Autodesk Inventor part; units mm, degrees
ref_plane "YZ Plane" through (0, 0, 0) normal (1, 0, 0) x (0, 1, 0)
ref_plane "XZ Plane" through (0, 0, 0) normal (0, 1, 0) x (-1, 0, 0)
ref_plane "XY Plane" through (0, 0, 0) normal (0, 0, 1) x (1, 0, 0)
sketch "Эскиз1" plane through (0, 0, 0) normal (0, 0, 1) x (1, 0, 0)
  line L0 (-30.974, -13.01) -> (30.974, -13.01)
  line L1 (30.974, -13.01) -> (30.974, 13.01)
  line L2 (30.974, 13.01) -> (-30.974, 13.01)
  line L3 (-30.974, 13.01) -> (-30.974, -13.01)
  line L4 (-30.974, -13.01) -> (30.974, 13.01) construction
  line L5 (30.974, -13.01) -> (-30.974, 13.01) construction
  point P0 (0, 0)
  dimension "d0" = 61.948
  dimension "d1" = 26.02
extrude "Выдавливание1" add sketch "Эскиз1" along normal blind 10
sketch "Эскиз2" plane through (30.974, -13.01, 0) normal (1, 0, 0) x (0, 0, -1)
  line L0 (0, 13.01) -> (-5, 13.01)
  circle A0 centre (-5, 13.01) radius 2
  dimension "d4" = 5
  dimension "d5" = 4
extrude "Выдавливание2" cut sketch "Эскиз2" against normal blind 10
pattern_linear "Прямоуг.массив1" count 3 spacing 8 along (0, 1, 0) of "Выдавливание2" first direction both ways yes
mirror "Зеркальное отражение1" about plane through (0, 0, 0) normal (1, 0, 0) of "Выдавливание2", "Прямоуг.массив1"
sketch "Эскиз3" plane through (0, 0, 0) normal (0, 0, -1) x (-1, 0, 0)
  line L0 (0, 0) -> (-20, 0)
  line L1 (-30.974, 13.01) -> (30.974, 13.01)
  line L2 (30.974, -13.01) -> (-30.974, -13.01)
  line L3 (-20, 13.01) -> (-25, 13.01)
  line L4 (-25, 13.01) -> (-25, -13.01)
  line L5 (-25, -13.01) -> (-20, -13.01)
  line L6 (-20, -13.01) -> (-20, 13.01)
  line L7 (-30.974, -13.01) -> (-30.974, 13.01)
  dimension "d11" = 20
  dimension "d12" = 5
extrude "Выдавливание3" add sketch "Эскиз3" along normal blind 10 contours L1 L6 L2 L4
sketch "Эскиз4" plane through (25, -13.01, 0) normal (1, 0, 0) x (0, 0, -1)
  line L0 (10, 26.02) -> (10, 0)
  line L1 (10, 13.01) -> (5, 13.01)
  circle A0 centre (5, 13.01) radius 2
  point P0 (0, 13.01)
  dimension "d16" = 5
  dimension "d17" = 4
extrude "Выдавливание4" cut sketch "Эскиз4" against normal blind 10
pattern_linear "Прямоуг.массив2" count 3 spacing 8 along (0, -1, 0) of "Выдавливание4" first direction both ways yes
mirror "Зеркальное отражение2" about plane through (0, 0, 0) normal (1, 0, 0) of "Выдавливание3", "Выдавливание4", "Прямоуг.массив2"
sketch "Эскиз5" plane through (0, 0, 10) normal (0, 0, 1) x (1, 0, 0)
  circle A0 centre (0, 0) radius 7.5
  dimension "d23" = 15
extrude "Выдавливание5" cut sketch "Эскиз5" against normal blind 23.75
sketch "Эскиз6" plane through (0, 0, 10) normal (0, 0, 1) x (1, 0, 0)
  circle A0 centre (0, 0) radius 5
  line L0 (-13.4261, 4.5029) -> (-16.9261, 4.5029)
  line L1 (-16.9261, 4.5029) -> (-16.9261, 11.4971)
  line L2 (-16.9261, 11.4971) -> (-13.4261, 11.4971)
  line L3 (-13.4261, 11.4971) -> (-13.4261, 4.5029)
  line L4 (-13.4261, -11.4971) -> (-16.9261, -11.4971)
  line L5 (-16.9261, -11.4971) -> (-16.9261, -4.5029)
  line L6 (-16.9261, -4.5029) -> (-13.4261, -4.5029)
  line L7 (-13.4261, -4.5029) -> (-13.4261, -11.4971)
  line L8 (-13.4261, -3.4971) -> (-16.9261, -3.4971)
  line L9 (-16.9261, -3.4971) -> (-16.9261, 3.4971)
  line L10 (-16.9261, 3.4971) -> (-13.4261, 3.4971)
  line L11 (-13.4261, 3.4971) -> (-13.4261, -3.4971)
  line L12 (10.5, 4.5029) -> (7, 4.5029)
  line L13 (7, 4.5029) -> (7, 11.4971)
  line L14 (7, 11.4971) -> (10.5, 11.4971)
  line L15 (10.5, 11.4971) -> (10.5, 4.5029)
  line L16 (10.5, -11.4971) -> (7, -11.4971)
  line L17 (7, -11.4971) -> (7, -4.5029)
  line L18 (7, -4.5029) -> (10.5, -4.5029)
  line L19 (10.5, -4.5029) -> (10.5, -11.4971)
  line L20 (7, 3.4971) -> (10.5, 3.4971)
  line L21 (10.5, 3.4971) -> (10.5, -3.4971)
  line L22 (10.5, -3.4971) -> (7, -3.4971)
  line L23 (7, -3.4971) -> (7, 3.4971)
  line L24 (17, -13.1) -> (17, 13.1)
  line L25 (17, 13.1) -> (-17, 13.1)
  line L26 (-17, 13.1) -> (-17, -13.1)
  line L27 (-17, -13.1) -> (17, -13.1)
extrude "Выдавливание6" cut sketch "Эскиз6" against normal blind 10 contours L0 L1 L2 L3 | L4 L5 L6 L7 | L8 L9 L10 L11
mirror "Зеркальное отражение3" about plane through (0, 0, 0) normal (1, 0, 0) of "Выдавливание6"
properties part number "000.404 - Переходник" material "Пластик АБС"
Work out the finished part from the listing and answer in its coordinate system (mm). A direction names the side the tool comes from. Coordinates: 2 decimals unless noted, no trailing zeros. Loops run counter-clockwise (first coordinate to the right, second up) from the corner with the lowest first, then second, coordinate; pieces in that order, holes last. Notation, with made-up numbers: (-24, -27.75) - (16, -27.75) arc R29 cw to (16, -3.75) - close; hole circle Ø9 at (81.5, 78). An arc over 180 degrees is marked (long way). Use a Markdown table: item, result.
Item 1: Find section B-B, the plane x = 0. Determine the outline of the cut face in (y, z).
Evaluation:
| item | result |
|---|---|
| outline | (-13.01, 0) - (-7.5, 0) - (-7.5, 10) - (-13.01, 10) - close; (7.5, 0) - (13.01, 0) - (13.01, 10) - (7.5, 10) - close |
Item 2: Find section A-A, the plane z = -5. State how many separate pieces and enclosed holes the cut face has, and give its area (3 significant figures).
Evaluation:
| item | result |
|---|---|
| separate pieces | 8 |
| enclosed holes | 0 |
| area | 140 mm2 |
Item 3: For faces 1 (the flat face through (0, 13.01, 4)), 2 (the flat face through (-20.974, 0, 5)), 3 (the flat face through (28, 0, 0)), 4 (the cylindrical face through (22.535, 9.352, -3.526)), 5 (the flat face through (13.426, 8, 5)), determine the directions among +Z, -Z, +X, -X, +Y, -Y from which every point of the face is accessible in a straight line to the end or side of a thin tool.
Evaluation:
| item | result |
|---|---|
| face 1 | +Z, -Z, +X, -X, +Y |
| face 2 | -X |
| face 3 | -Z, +X, +Y, -Y |
| face 4 | +X, -X |
| face 5 | +Z, -Z |
Item 4: The mould has two halves that part along X. Classify faces 6 (the flat face through (-13.426, 8, 5)), 7 (the flat face through (-20.974, 8, 5)), 8 (the flat face through (16.926, 0, 5)), 9 (the flat face through (6, 6, 10)): +X half, -X half, draft (parallel to the pull), parting line (faces both ways), or undercut.
Evaluation:
| item | result |
|---|---|
| face 6 | undercut |
| face 7 | -X half |
| face 8 | undercut |
| face 9 | draft |
Item 5: Given pin 1 Ø13 at (x, y) = (-7, 2.5) entering from -Z; pin 2 Ø3 at (y, z) = (-8, 5) entering from +X; pin 3 Ø6.5 at (y, z) = (0, -5) entering from -X, each flat-ended and moving along its own axis, determine where each tip first touches the part or whether it passes through.
Evaluation:
| item | result |
|---|---|
| pin 1 | stops at z = 0 |
| pin 2 | stops at x = 20.97 |
| pin 3 | stops at x = -25 |
Item 6: Consider probe 1 along Y at (x, z) = (-26, 5); probe 2 along X at (y, z) = (-10.75, 7.75); probe 3 along X at (y, z) = (-10.5, -0.5). Determine where each line is inside the solid, lowest interval first. Write a range as from..to.
Evaluation:
| item | result |
|---|---|
| probe 1 | y = -13.01..-10, -6..-2, 2..6, 10..13.01 |
| probe 2 | x = -30.97..-16.93, -13.43..13.43, 16.93..30.97 |
| probe 3 | x = -25..-20, 20..25 |
